Check sheet for the modelled part. Datum: model origin and axes. Units: mm. Face numbers are marked on the shaded views. A direction names the side the tool comes from. Round coordinates to 2 decimals unless told otherwise and drop trailing zeros. Loops run counter-clockwise (first coordinate to the right, second up) from the corner with the lowest first, then second, coordinate; pieces in that order, holes last. Notation, with made-up numbers: (22.25, 70) -> (63.25, 70) arc R19 cw to (63.25, 103) -> close; hole circle Ø1 at (55.5, 14). An arc over 180 degrees is marked (long way). One line per item, written item: value. Start each with the question number.
1. Cross-section at A-A on y = -1.25. Record the cut outline in (x, z).
2. Cross-section at D-D on z = -0.5. Record the cut outline in (x, y), then the cut area to 3 significant figures.
3. Cross-section at B-B on x = -10.75. Record the cut outline in (y, z).
4. Go/stop test with flat-tipped pins: pin 1 (3 mm diameter, centred on x = 10, z = 1, fed in from -Y); pin 2 (6 mm diameter, centred on x = -8, y = -13, fed in from -Z); pin 3 (6 mm diameter, centred on y = -14.5, z = 2.5, fed in from +X); pin 4 (1.8 mm diameter, centred on x = -1.5, z = -1.5, fed in from -Y). Record where each tip stops, or that it passes through.
5. Release check for a two-part mould opening along Z. For the marked faces 4, 5 and 6 record: +Z half, -Z half, draft (parallel to the pull), parting line (faces both ways), or undercut.
6. Cross-section at C-C on z = -2.5. Record the cut outline in (x, y), then the cut area to 3 significant figures.
7. Material ranges on L1, parallel to Z at x = -10, y = -3.75; L2, parallel to X at y = -17, z = -0.5; L3, parallel to Y at x = 7, z = 2.5, recorded low to high.
8. Set-up check for the marked faces 1, 2 and 3: record each of +Z, -Z, +X, -X, +Y, -Y from which the full face is reachable in a straight line by a thin tool's end or side.
from build123d import *

# Parameters (mm, degrees)
F0_W      = 30
F0_H      = 12
F1_DEPTH  = 6
F2_W      = 10
F2_H      = 12
F3_DEPTH  = 4
F4_W      = 1.5
F4_H      = 12
F5_DEPTH  = 8
F6_SIZE   = 2
F7_SIZE   = 0.5
F10_DEPTH = 6
F12_DEPTH = 6


with BuildPart() as f1:
    # F0 (on Front) → F1 (new body)
    with BuildSketch(Plane.XZ):
        Rectangle(F0_W, F0_H)
    extrude(amount=F1_DEPTH)

    # F2 (on face) → F3 (join)
    with BuildSketch(Plane.XZ.offset(6)):
        Rectangle(F2_W, F2_H)
    extrude(amount=F3_DEPTH)

    # F4 (on face) → F5 (join)
    with BuildSketch(Plane.XZ.offset(10)):
        Rectangle(F4_W, F4_H)
    extrude(amount=F5_DEPTH)

    # F6
    f6_edges = [f1.edges().sort_by_distance(p)[0] for p in [
        (-5, -10, 0),
        (5, -10, 0),
    ]]
    chamfer(f6_edges, length=F6_SIZE)

    # F7
    f7_edges = [f1.edges().sort_by_distance(p)[0] for p in [
        (-0.75, -18, 0),
        (0.75, -18, 0),
    ]]
    chamfer(f7_edges, length=F7_SIZE)

    # F9 (on face) → F10 (cut, through all)
    with BuildSketch(Plane.XZ.offset(6)):
        with BuildLine():
            Line((8.028282, 1.499733), (7.971718, 1.499733))
            ThreePointArc((7.971718, 1.499733), (6.500096, -0.016942), (8.005601, -1.49999))
            ThreePointArc((8.005601, -1.49999), (9.062639, -1.058678), (9.5, 0))
            ThreePointArc((9.5, 0), (9.070613, 1.050614), (8.028282, 1.499733))
        make_face()
        with BuildLine():
            ThreePointArc((8.028282, 1.499733), (8, 1.5), (7.971718, 1.499733))
            Line((7.971718, 1.499733), (8.028282, 1.499733))
        make_face()
        with BuildLine():
            ThreePointArc((9.5, 0), (9.062639, -1.058678), (8.005601, -1.49999))
            Line((8.005601, -1.49999), (11.999996, -1.5))
            ThreePointArc((11.999996, -1.5), (10.500067, -0.014139), (11.971718, 1.499733))
            Line((11.971718, 1.499733), (8.028282, 1.499733))
            ThreePointArc((8.028282, 1.499733), (9.070613, 1.050614), (9.5, 0))
        make_face()
        with BuildLine():
            ThreePointArc((11.971718, 1.499733), (10.500067, -0.014139), (11.999996, -1.5))
            ThreePointArc((11.999996, -1.5), (13.060659, -1.060662), (13.5, 0))
            ThreePointArc((13.5, 0), (13.050614, 1.070613), (11.971718, 1.499733))
        make_face()
    extrude(amount=-F10_DEPTH, mode=Mode.SUBTRACT)

    # F11 (on face) → F12 (cut, through all)
    with BuildSketch(Plane.XZ.offset(6)):
        with BuildLine():
            Line((-11.948695, 1.499122), (-12.051971, 1.499099))
            ThreePointArc((-12.051971, 1.499099), (-13.499095, -0.052084), (-11.947804, -1.499092))
            ThreePointArc((-11.947804, -1.499092), (-10.921043, -1.042043), (-10.5, 0))
            ThreePointArc((-10.5, 0), (-10.921353, 1.042363), (-11.948695, 1.499122))
        make_face()
        with BuildLine():
            ThreePointArc((-11.948695, 1.499122), (-12.000333, 1.5), (-12.051971, 1.499099))
            Line((-12.051971, 1.499099), (-11.948695, 1.499122))
        make_face()
        with BuildLine():
            ThreePointArc((-10.5, 0), (-10.921043, -1.042043), (-11.947804, -1.499092))
            Line((-11.947804, -1.499092), (-8.000345, -1.5))
            ThreePointArc((-8.000345, -1.5), (-9.5, 6e-06), (-8.000333, 1.5))
            Line((-8.000333, 1.5), (-11.948695, 1.499122))
            ThreePointArc((-11.948695, 1.499122), (-10.921353, 1.042363), (-10.5, 0))
        make_face()
        with BuildLine():
            ThreePointArc((-8.000333, 1.5), (-9.5, 6e-06), (-8.000345, -1.5))
            ThreePointArc((-8.000345, -1.5), (-6.939462, -1.060782), (-6.5, 0))
            ThreePointArc((-6.5, 0), (-6.939458, 1.060778), (-8.000333, 1.5))
        make_face()
    extrude(amount=-F12_DEPTH, mode=Mode.SUBTRACT)


solid = f1.part
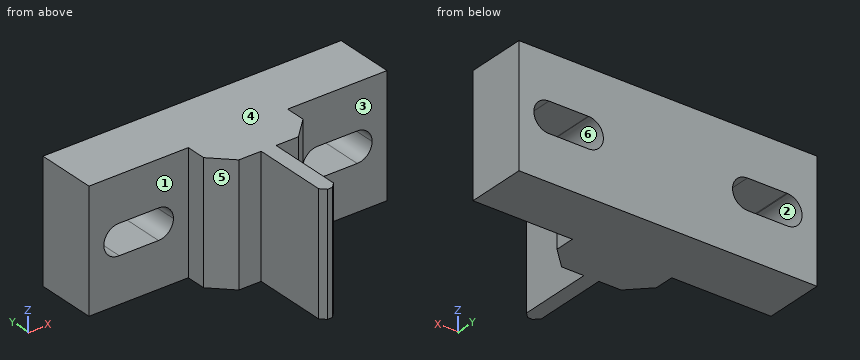
Taken from the geometry:
1. outline: (-15, -6) -> (15, -6) -> (15, 6) -> (-15, 6) -> close; hole (-12.05, 1.5) arc R1.5 ccw to (-11.95, -1.5) -> (-8, -1.5) arc R1.5 ccw to (-6.5, 0) arc R1.5 ccw to (-8, 1.5) -> (-11.95, 1.5) arc R1.5 ccw to start; hole (7.97, 1.5) arc R1.5 ccw to (8.01, -1.5) -> (12, -1.5) arc R1.5 ccw to (13.5, 0) arc R1.5 ccw to (11.97, 1.5) -> (8.03, 1.5) arc R1.5 ccw to start
2. outline: (-15, -6) -> (-13.41, -6) -> (-13.41, 0) -> (-15, 0) -> close; (-6.59, -6) -> (-5, -6) -> (-5, -8) -> (-3, -10) -> (-0.75, -10) -> (-0.75, -17.5) -> (-0.25, -18) -> (0.25, -18) -> (0.75, -17.5) -> (0.75, -10) -> (3, -10) -> (5, -8) -> (5, -6) -> (6.59, -6) -> (6.59, 0) -> (-6.59, 0) -> close; (13.41, -6) -> (15, -6) -> (15, 0) -> (13.41, 0) -> close
2. area: 146 mm2
3. outline: (-6, -6) -> (0, -6) -> (0, -1.5) -> (-6, -1.5) -> close; (-6, 1.5) -> (0, 1.5) -> (0, 6) -> (-6, 6) -> close
4. pin 1: stops at y = -6
4. pin 2: passes through
4. pin 3: stops at x = 0.75
4. pin 4: stops at y = -17.65
5. face 4: +Z half
5. face 5: draft
5. face 6: undercut
6. outline: (-15, -6) -> (-5, -6) -> (-5, -8) -> (-3, -10) -> (-0.75, -10) -> (-0.75, -17.5) -> (-0.25, -18) -> (0.25, -18) -> (0.75, -17.5) -> (0.75, -10) -> (3, -10) -> (5, -8) -> (5, -6) -> (15, -6) -> (15, 0) -> (-15, 0) -> close
6. area: 228 mm2
7. L1: z = -6 to -1.5, 1.5 to 6
7. L2: x = -0.75 to 0.75
7. L3: y = -6 to 0
8. face 1: +Z, -Z, -X, -Y
8. face 2: +Y, -Y
8. face 3: +Z, -Z, +X, -Y
